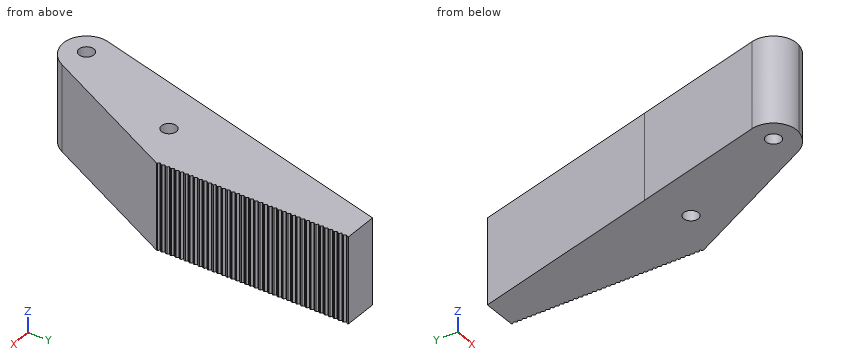
from build123d import *

# Parameters (mm, degrees)
F1_DEPTH = 19.05
F3_DEPTH = 19.05
F4_R     = 5.08
F5_R     = 1.651
F6_DEPTH = 19.05
F8_DEPTH = 19.051


with BuildPart() as f1:
    # F0 (on Top) → F1 (new body)
    with BuildSketch(Plane.XY):
        with BuildLine():
            Line((2.7951651794, -31.627423938), (19.05, 0))
            Line((19.05, 0), (19.05, 63.5))
            Line((19.05, 63.5), (17.4625, 63.5))
            Line((17.4625, 63.5), (0, 0))
            Line((0, 0), (-8.9422228719, -32.5171740795))
            ThreePointArc((-8.9422228719, -32.5171740795), (-2.8245693117, -35.3565183974), (2.7951651794, -31.627423938))
        make_face()
    extrude(amount=F1_DEPTH)

    # F2 (on face) → F3 (cut, through all)
    with BuildSketch(Plane.XY.offset(19.05)):
        Polygon((18.7139895835, 0.635), (19.05, 0.254), (19.05, 1.016), align=None)
        Polygon((19.05, 2.032), (18.7139895835, 1.651), (19.05, 1.27), align=None)
        Polygon((19.05, 3.048), (18.7139895835, 2.667), (19.05, 2.286), align=None)
        Polygon((19.05, 4.064), (18.7139895835, 3.683), (19.05, 3.302), align=None)
        Polygon((19.05, 5.08), (18.7139895835, 4.699), (19.05, 4.318), align=None)
        Polygon((19.05, 6.096), (18.7139895835, 5.715), (19.05, 5.334), align=None)
        Polygon((19.05, 7.112), (18.7139895835, 6.731), (19.05, 6.35), align=None)
        Polygon((19.05, 8.128), (18.7139895835, 7.747), (19.05, 7.366), align=None)
        Polygon((19.05, 9.144), (18.7139895835, 8.763), (19.05, 8.382), align=None)
        Polygon((19.05, 10.16), (18.7139895835, 9.779), (19.05, 9.398), align=None)
        Polygon((19.05, 11.176), (18.7139895835, 10.795), (19.05, 10.414), align=None)
        Polygon((19.05, 12.192), (18.7139895835, 11.811), (19.05, 11.43), align=None)
        Polygon((19.05, 13.208), (18.7139895835, 12.827), (19.05, 12.446), align=None)
        Polygon((19.05, 14.224), (18.7139895835, 13.843), (19.05, 13.462), align=None)
        Polygon((19.05, 15.24), (18.7139895835, 14.859), (19.05, 14.478), align=None)
        Polygon((19.05, 16.256), (18.7139895835, 15.875), (19.05, 15.494), align=None)
        Polygon((19.05, 17.272), (18.7139895835, 16.891), (19.05, 16.51), align=None)
        Polygon((19.05, 18.288), (18.7139895835, 17.907), (19.05, 17.526), align=None)
        Polygon((19.05, 19.304), (18.7139895835, 18.923), (19.05, 18.542), align=None)
        Polygon((19.05, 20.32), (18.7139895835, 19.939), (19.05, 19.558), align=None)
        Polygon((19.05, 21.336), (18.7139895835, 20.955), (19.05, 20.574), align=None)
        Polygon((19.05, 22.352), (18.7139895835, 21.971), (19.05, 21.59), align=None)
        Polygon((19.05, 23.368), (18.7139895835, 22.987), (19.05, 22.606), align=None)
        Polygon((19.05, 24.384), (18.7139895835, 24.003), (19.05, 23.622), align=None)
        Polygon((19.05, 25.4), (18.7139895835, 25.019), (19.05, 24.638), align=None)
        Polygon((19.05, 26.416), (18.7139895835, 26.035), (19.05, 25.654), align=None)
        Polygon((19.05, 27.432), (18.7139895835, 27.051), (19.05, 26.67), align=None)
        Polygon((19.05, 28.448), (18.7139895835, 28.067), (19.05, 27.686), align=None)
        Polygon((19.05, 29.464), (18.7139895835, 29.083), (19.05, 28.702), align=None)
        Polygon((19.05, 30.48), (18.7139895835, 30.099), (19.05, 29.718), align=None)
        Polygon((19.05, 31.496), (18.7139895835, 31.115), (19.05, 30.734), align=None)
        Polygon((19.05, 32.512), (18.7139895835, 32.131), (19.05, 31.75), align=None)
        Polygon((19.05, 33.528), (18.7139895835, 33.147), (19.05, 32.766), align=None)
        Polygon((19.05, 34.544), (18.7139895835, 34.163), (19.05, 33.782), align=None)
        Polygon((19.05, 35.56), (18.7139895835, 35.179), (19.05, 34.798), align=None)
        Polygon((19.05, 36.576), (18.7139895835, 36.195), (19.05, 35.814), align=None)
        Polygon((19.05, 37.592), (18.7139895835, 37.211), (19.05, 36.83), align=None)
        Polygon((19.05, 38.608), (18.7139895835, 38.227), (19.05, 37.846), align=None)
        Polygon((19.05, 39.624), (18.7139895835, 39.243), (19.05, 38.862), align=None)
        Polygon((19.05, 40.64), (18.7139895835, 40.259), (19.05, 39.878), align=None)
        Polygon((19.05, 41.656), (18.7139895835, 41.275), (19.05, 40.894), align=None)
        Polygon((19.05, 42.672), (18.7139895835, 42.291), (19.05, 41.91), align=None)
        Polygon((19.05, 43.688), (18.7139895835, 43.307), (19.05, 42.926), align=None)
        Polygon((19.05, 44.704), (18.7139895835, 44.323), (19.05, 43.942), align=None)
        Polygon((19.05, 45.72), (18.7139895835, 45.339), (19.05, 44.958), align=None)
        Polygon((19.05, 46.736), (18.7139895835, 46.355), (19.05, 45.974), align=None)
        Polygon((19.05, 47.752), (18.7139895835, 47.371), (19.05, 46.99), align=None)
        Polygon((19.05, 48.768), (18.7139895835, 48.387), (19.05, 48.006), align=None)
        Polygon((19.05, 49.784), (18.7139895835, 49.403), (19.05, 49.022), align=None)
        Polygon((19.05, 50.8), (18.7139895835, 50.419), (19.05, 50.038), align=None)
        Polygon((19.05, 51.816), (18.7139895835, 51.435), (19.05, 51.054), align=None)
        Polygon((19.05, 52.832), (18.7139895835, 52.451), (19.05, 52.07), align=None)
        Polygon((19.05, 53.848), (18.7139895835, 53.467), (19.05, 53.086), align=None)
        Polygon((19.05, 54.864), (18.7139895835, 54.483), (19.05, 54.102), align=None)
        Polygon((19.05, 55.88), (18.7139895835, 55.499), (19.05, 55.118), align=None)
        Polygon((19.05, 56.896), (18.7139895835, 56.515), (19.05, 56.134), align=None)
        Polygon((19.05, 57.912), (18.7139895835, 57.531), (19.05, 57.15), align=None)
        Polygon((19.05, 58.928), (18.7139895835, 58.547), (19.05, 58.166), align=None)
        Polygon((19.05, 59.944), (18.7139895835, 59.563), (19.05, 59.182), align=None)
        Polygon((19.05, 60.96), (18.7139895835, 60.579), (19.05, 60.198), align=None)
        Polygon((19.05, 61.976), (18.7139895835, 61.595), (19.05, 61.214), align=None)
        Polygon((19.05, 62.992), (18.7139895835, 62.611), (19.05, 62.23), align=None)
    extrude(amount=-F3_DEPTH, mode=Mode.SUBTRACT)

    # F4
    f4_edges = [f1.edges().sort_by_distance(p)[0] for p in [
        (-8.942223, -32.517174, 9.525),
    ]]
    fillet(f4_edges, radius=F4_R)

    # F5 (on face) → F6 (cut, through all)
    with BuildSketch(Plane.XY.offset(19.05)):
        with Locations((-3.0565118627, -30.2730867816)):
            Circle(F5_R)
        with Locations((8.7544881373, -4.2380867816)):
            Circle(F5_R)
    extrude(amount=-F6_DEPTH, mode=Mode.SUBTRACT)

    # F7 (on face) → F8 (cut, through all)
    with BuildSketch(Plane.XY.offset(19.05)):
        Polygon((19.05, 63.5), (17.4625, 63.5), (11.5776375, 42.1005), (19.05, 41.91), align=None)
    extrude(amount=-F8_DEPTH, mode=Mode.SUBTRACT)


solid = f1.part
Part model, mm, in its own coordinate system. Coordinates: 2 decimals unless noted, no trailing zeros. Order: outer loops, then holes, each group sorted by start corner. A loop starts at its lowest first (then second) coordinate and runs counter-clockwise, first axis right, second up.
(1) Slice it at B-B, the plane z = 4.5. State how many separate pieces and enclosed holes the cut face has, and give its area (3 significant figures).
Check sheet entries:
separate pieces: 1
enclosed holes: 2
area: 1,050 mm2
(2) Pin check, flat tips, straight feed: pin 1 Ø1 at (y, z) = (6.5, 15.5) entering from -X; pin 2 Ø2 at (x, y) = (8.75, -4.24) entering from -Z; pin 3 Ø6 at (y, z) = (22.5, 6.5) entering from -X; pin 4 Ø10 at (y, z) = (-6, 3.5) entering from -X (3 decimals). Stop position of each tip, or through.
Check sheet entries:
pin 1: stops at x = 1.65
pin 2: passes through
pin 3: stops at x = 5.36
pin 4: stops at x = -3.025
(3) Slice it at C-C, the plane x = 15.5. Write the cut outline in (y, z).
Check sheet entries:
outline: (-6.91, 0) - (42, 0) - (42, 19.05) - (-6.91, 19.05) - close
(4) Probe L1, parallel to X at y = -26, z = 16.5; L2, parallel to Y at x = 18, z = 3; L3, parallel to X at y = -18, z = 13.5. List the from-to ranges inside material, lowest first.
Check sheet entries:
L1: x = -7.15 to 5.69
L2: y = -2.04 to 41.94
L3: x = -4.95 to 9.8
(5) Slice it at D-D, the plane y = -8. Write the cut outline in (x, z).
Check sheet entries:
outline: (-2.2, 0) - (14.94, 0) - (14.94, 19.05) - (-2.2, 19.05) - close
(6) Slice it at A-A, the plane x = 9.5. Write the cut outline in (y, z) (3 decimals), and give its area (3 significant figures).
Check sheet entries:
outline: (-18.582, 0) - (-5.711, 0) - (-5.711, 19.05) - (-18.582, 19.05) - close; (-2.765, 0) - (34.545, 0) - (34.545, 19.05) - (-2.765, 19.05) - close
area: 956 mm2
